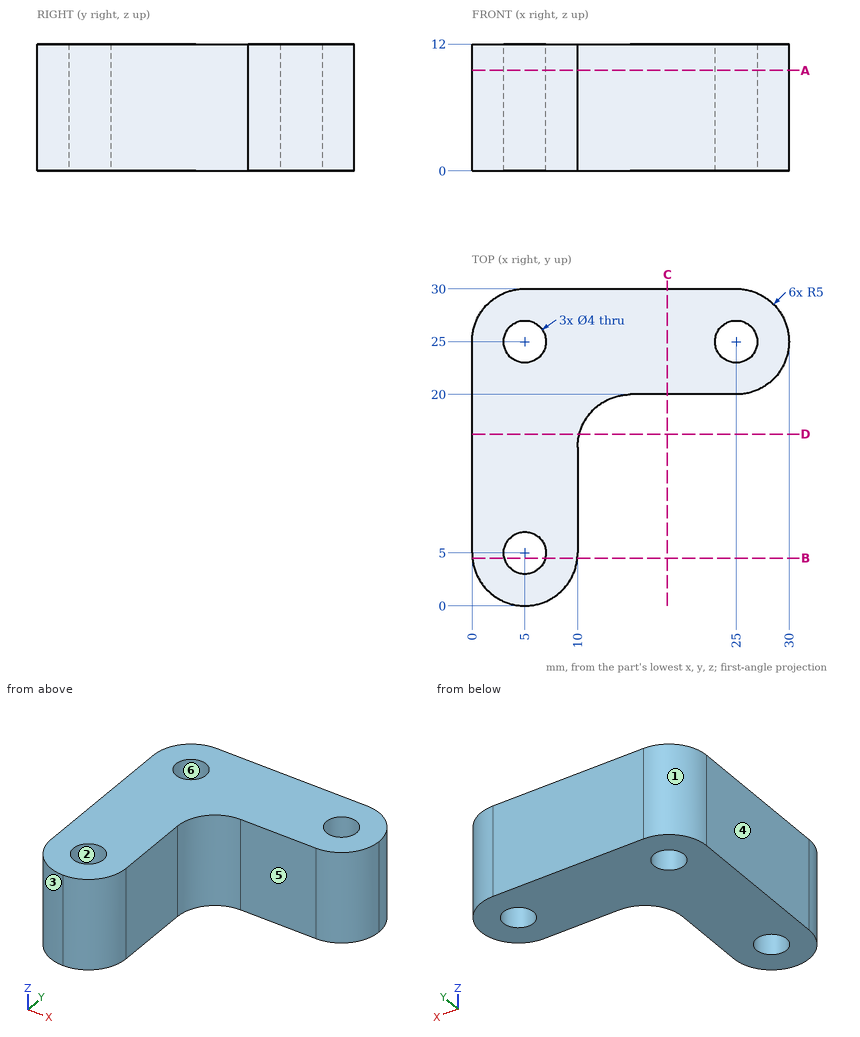
Part print with two shaded views. Sizes in mm from the minimum x, y, z corner. A direction names the side the tool comes from. Round coordinates to 2 decimals unless told otherwise and drop trailing zeros. Loops run counter-clockwise (first coordinate to the right, second up) from the corner with the lowest first, then second, coordinate; pieces in that order, holes last. Notation, with made-up numbers: (39, 22) - (45, 22) arc R33 cw to (45, 60) - close; hole circle Ø10 at (72, 78). An arc over 180 degrees is marked (long way). Put each result on its own line as item: value.
1. Slice it at B-B on y = 4.5. List the corners of the cut face in (x, z) (1 decimal), and give its area (3 significant figures).
Geometry check:
outline: (0, 0) - (3.1, 0) - (3.1, 12) - (0, 12) - close; (6.9, 0) - (10, 0) - (10, 12) - (6.9, 12) - close
area: 72.9 mm²
2. Two-plate mould, pull along Y, no slides. Class the marked faces 1, 2, 3 and 4: released by +Y, released by -Y, zero draft, split by the parting line, or undercut.
Geometry check:
face 1: released by +Y
face 2: undercut
face 3: released by -Y
face 4: zero draft
3. Slice it at D-D on y = 16.25. List the corners of the cut face in (x, z).
Geometry check:
outline: (0, 0) - (10.16, 0) - (10.16, 12) - (0, 12) - close
4. Pin check, flat tips, straight feed: P1, Ø2, axis at y = 6.5, z = 4.5, coming from the +X side; P2, Ø3, axis at x = 19, z = 9, coming from the -Y side; P3, Ø6, axis at y = 20, z = 3.5, coming from the +X side. Stop position of each tip, or through.
Geometry check:
P1: x = 10
P2: y = 20
P3: x = 29.58
5. Slice it at A-A on z = 9.5. Give the number of separate pieces and of enclosed holes in the cut face, and give its area (3 significant figures).
Geometry check:
separate pieces: 1
enclosed holes: 3
area: 441 mm²
6. Slice it at C-C on x = 18.5. List the corners of the cut face in (y, z), and give its area (3 significant figures).
Geometry check:
outline: (20, 0) - (30, 0) - (30, 12) - (20, 12) - close
area: 120 mm²
7. 3-axis set-ups, long thin cutter, end or side, ignore diameter. For the marked faces 5 and 6: which of +Z, -Z, +X, -X, +Y, -Y reach the whole face in a straight line?
Geometry check:
face 5: +Z, -Z, +X, -Y
face 6: +Z, -Z
8. Wall check: line 1 (Y direction, x = 5, z = 3.5); line 2 (Y direction, x = 25, z = 6); line 3 (X direction, y = 11.75, z = 6.25). Give the ranges that are in metal, low to high.
Geometry check:
line 1: 0 to 3, 7 to 23, 27 to 30
line 2: 20 to 23, 27 to 30
line 3: 0 to 10
